from build123d import *

# Parameters (mm, degrees)
SKETCH014_W     = 15
SKETCH014_H     = 65
PAD008_DEPTH    = 15
SKETCH015_R     = 2
POCKET005_DEPTH = 4
SKETCH016_R     = 2
POCKET006_DEPTH = 4


with BuildPart() as part:
    # Sketch014 → Pad008 (new body)
    with BuildSketch(Plane(origin=(-27, 0, 50), x_dir=(1, 0, 0), z_dir=(0, 0, 1))):
        with Locations((-7.5, 0)):
            Rectangle(SKETCH014_W, SKETCH014_H)
    extrude(amount=-PAD008_DEPTH)

    # Sketch015 → Pocket005 (cut)
    with BuildSketch(Plane(origin=(-34.5, 0, 50), x_dir=(1, 0, 0), z_dir=(0, 0, 1))):
        with Locations((0, 23.75)):
            Circle(SKETCH015_R)
        with Locations((0, -23.75)):
            Circle(SKETCH015_R)
    extrude(amount=-POCKET005_DEPTH, mode=Mode.SUBTRACT)

    # Sketch016 → Pocket006 (cut)
    with BuildSketch(Plane.YZ.offset(-27)):
        with Locations((-9.5, 42.5)):
            Circle(SKETCH016_R)
        with Locations((9.5, 42.5)):
            Circle(SKETCH016_R)
    extrude(amount=-POCKET006_DEPTH, mode=Mode.SUBTRACT)


solid = part.part
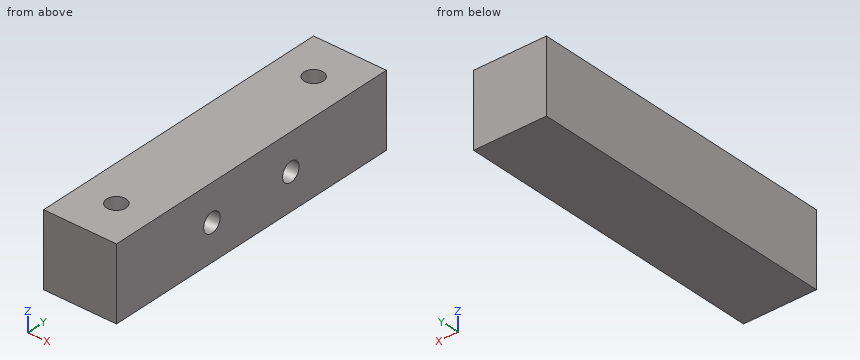
Design review of the part built by this model. Coordinates are the model's own, in mm. Round coordinates to 2 decimals unless told otherwise and drop trailing zeros. Write each loop counter-clockwise with the first axis right and the second up, starting at its lowest first coordinate (ties: lowest second). Pieces come first, ordered by that corner, then holes. Notation, with made-up numbers: (-14.5, 57) - (27.5, 57) arc R18 cw to (27.5, 75) - close; hole circle Ø3 at (89.5, 31). An arc over 180 degrees is marked (long way). Return JSON: item names as keys, results as strings. Group by question number.
Item 1: We need section C-C on x = -34.5. Write out the cut boundary in (y, z), and give its area (3 significant figures).
Item 2: We need section B-B on y = -23.75. Write out the cut boundary in (x, z).
Item 3: We need section A-A on x = -28.25. Write out the cut boundary in (y, z), and give its area (3 significant figures).
Item 4: For probe 1 along Y at (x, z) = (-34.5, 47.45); probe 2 along Z at (x, y) = (-29.4, 9.5); probe 3 along X at (y, z) = (-9, 40.75), list the stretches that pass through material, from the lowest coordinate up. Write a range as [from, to].
Item 5: Insertion check: P1, Ø2, axis at x = -34.5, y = 24, coming from the +Z side; P2, Ø1.2, axis at y = 9.5, z = 43, coming from the +X side. Each pin has a flat end and moves straight along its axis. Give the tip position at first contact, or say it passes through.
Item 6: We need section D-D on z = 49.25. Write out the cut boundary in (x, y).
Model answer:
{
 "1": {"outline": "(-32.5, 35) - (32.5, 35) - (32.5, 50) - (25.75, 50) - (25.75, 46) - (21.75, 46) - (21.75, 50) - (-21.75, 50) - (-21.75, 46) - (-25.75, 46) - (-25.75, 50) - (-32.5, 50) - close", "area": "943 mm²"},
 "2": {"outline": "(-42, 35) - (-27, 35) - (-27, 50) - (-32.5, 50) - (-32.5, 46) - (-36.5, 46) - (-36.5, 50) - (-42, 50) - close"},
 "3": {"outline": "(-32.5, 35) - (32.5, 35) - (32.5, 50) - (-32.5, 50) - close; hole circle Ø4 at (-9.5, 42.5); hole circle Ø4 at (9.5, 42.5)", "area": "950 mm²"},
 "4": {"probe 1": "y = [-32.5, -25.75], [-21.75, 21.75], [25.75, 32.5]", "probe 2": "z = [35, 40.5], [44.5, 50]", "probe 3": "x = [-42, -31]"},
 "5": {"P1": "stops at z = 46", "P2": "stops at x = -31"},
 "6": {"outline": "(-42, -32.5) - (-27, -32.5) - (-27, 32.5) - (-42, 32.5) - close; hole circle Ø4 at (-34.5, -23.75); hole circle Ø4 at (-34.5, 23.75)"}
}
